```python
from build123d import *

# Parameters (mm, degrees)
ESQUISSE5_R             = 1
ENL_V_MAT_EXTRU_2_DEPTH = 10


with BuildPart() as part:
    # Esquisse1 → Révolution2 (revolve)
    with BuildSketch(Plane.XY):
        with BuildLine():
            Line((0, 5), (0, -5))
            Line((0, -5), (-2.2, -5))
            ThreePointArc((-2.2, -5), (-1.357495617, -3.68245461), (-1.5, -2.125074762))
            ThreePointArc((-1.5, -2.125074762), (-1.747791972, -1.637919756), (-2.042253504, -1.177470772))
            ThreePointArc((-2.042253504, -1.177470772), (-2.5, 0), (-2.042253504, 1.177470772))
            ThreePointArc((-2.042253504, 1.177470772), (-1.747791972, 1.637919756), (-1.5, 2.125074762))
            ThreePointArc((-1.5, 2.125074762), (-1.357495617, 3.68245461), (-2.2, 5))
            Line((-2.2, 5), (0, 5))
        make_face()
    revolve(axis=Axis((0, -2, 0), (0, -1, 0)))

    # Esquisse5 → Enlèv. mat.-Extru.2 (cut)
    with BuildSketch(Plane(origin=(0, -5, 0), x_dir=(-1, 0, 0), z_dir=(0, -1, 0))):
        with Locations(Location((0, 0, 0), (0, 0, 180))):
            Circle(ESQUISSE5_R)
    extrude(amount=-ENL_V_MAT_EXTRU_2_DEPTH, mode=Mode.SUBTRACT)


solid = part.part
```
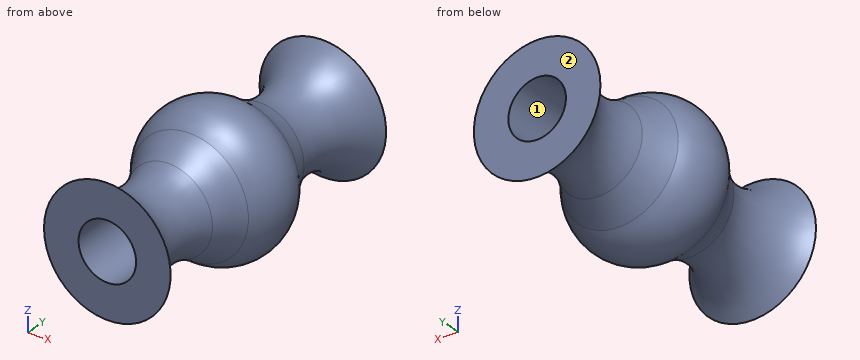
Input: part model. Units: mm. Frame: model coordinates. Face numbers are marked on the shaded views. Round coordinates to 2 decimals unless told otherwise and drop trailing zeros. One line per item, written item: value. Start each with the question number.
(1) Ray query, line 1 (Z direction, x = 0, y = 2.5); line 2 (Z direction, x = 0.2, y = 1.25); line 3 (X direction, y = -1.5, z = 0.4). Return the intervals inside material, ascending. Write a range as [from, to].
(2) Draft query along X for the marked faces 1 and 2. Return one class per face: +X half, -X half, draft (parallel to the pull), parting line (faces both ways), or undercut.
(3) Section A-A, the plane z = 1.65. Count the separate pieces of the cut face and the enclosed holes in it, plus the area to 3 significant figures.
(4) Contact query for flat-ended pins moving along their axis: P1, Ø2.5, axis at x = 0, z = 0, coming from the -Y side; P2, Ø2, axis at y = 1.5, z = 1.5, coming from the +X side; P3, Ø3, axis at x = 0.5, y = -3, coming from the +Z side; P4, Ø1, axis at x = 1, y = -3, coming from the +Z side. Output: stop coordinate, or through.
Results below:
1. line 1: [-1.37, -1], [1, 1.37]
1. line 2: [-1.98, -0.98], [0.98, 1.98]
1. line 3: [-1.79, -0.92], [0.92, 1.79]
2. face 1: undercut
2. face 2: draft
3. separate pieces: 3
3. enclosed holes: 0
3. area: 12.0 mm^2
4. P1: y = -5
4. P2: x = 2.18
4. P3: z = 1.8
4. P4: z = 1.19
